For this review, take the finished solid that the model builds, in its own axes (mm). A direction names the side the tool comes from. Coordinates: 2 decimals unless noted, no trailing zeros. Order: outer loops, then holes, each group sorted by start corner. A loop starts at its lowest first (then second) coordinate and runs counter-clockwise, first axis right, second up. Notation, with made-up numbers: (51.5, 77.25) -> (87.5, 77.25) arc R19 ccw to (87.5, 108.25) -> close; hole circle Ø7 at (55, 85). An arc over 180 degrees is marked (long way). Return JSON: item names as keys, results as strings. Group by question number.
Item 1: Draft analysis for pull direction Y (two halves, no side actions). For faces 1 (the cylindrical face through (187.95, 4.47, -0.06)), 2 (the flat face through (101.23, 8.06, -0.42)), 3 (the flat face through (179.43, -2.385, -0.056)), state which applies: +Y half, -Y half, draft (parallel to the pull), parting line (faces both ways), or undercut.
Item 2: Machinability: for faces 4 (the flat face through (156, 54, 4)), 5 (the flat face through (192.854, 51, 0)), 6 (the flat face through (119.747, 51, 0)), 7 (the flat face through (99.28, -36.72, -0.06)), which of the approach directions +Z, -Z, +X, -X, +Y, -Y give a long, thin tool a straight path to every point of the face, cutting with its end or side? Answer none if there is none.
Item 3: Insertion check: pin 1 (1.5 mm diameter, centred on x = 123.5, z = -14, fed in from -Y); pin 2 (8 mm diameter, centred on x = 128.17, y = -49.49, fed in from +Z); pin 3 (11 mm diameter, centred on x = 166.5, y = 54, fed in from -Z); pin 4 (4.5 mm diameter, centred on x = 136.48, y = 50.87, fed in from -Z). Each pin has a flat end and moves straight along its axis. Give the tip position at first contact, or say it passes through.
Item 4: For line 1 along Z through (x, y) = (215.5, 24); line 2 along Y through (x, z) = (108, -22.5); line 3 along Y through (x, z) = (226, 21), list the stretches that pass through material, from the lowest coordinate up.
Item 5: Take a section at A-A (y = -10.5). Write out the cut boundary in (x, z).
```python
from build123d import *

# Parameters (mm, degrees)
RIGHT_MAIN_DEPTH    = 30
SKETCH2_R           = 2.5625
SKETCH2_R_2         = 2.563
RIGHTSCREWS_DEPTH   = 4
LEFT_MAIN_START     = -30
LEFT_MAIN_DEPTH     = 30
BOSS_EXTRUDE4_START = -4
LEFTSCRWS_R         = 2.5625
LEFTSCRWS_R_2       = 2.563
BOSS_EXTRUDE4_DEPTH = 4


with BuildPart() as part:
    # Sketch1 → right_main (new body)
    with BuildSketch(Plane.XY):
        with BuildLine():
            Line((107.405043491, 43.874842), (94.874715104, -28.778692489))
            add(Edge.make_bspline(
                [(94.874715104, -28.778692489), (125.81929731, -36.765852729), (149.855864514, -58.067716007)],
                knots=[0, 0, 0, 1, 1, 1], degree=2))
            Line((149.855864514, -58.067716007), (149.855864514, 43.874842))
            Line((149.855864514, 43.874842), (107.405043491, 43.874842))
        make_face()
        Polygon((149.855864514, 43.874842), (149.855864514, 28.52351163), (234.383754043, 28.52351163), (234.383754043, 43.874842), (192.853964769, 43.874842), align=None)
        with BuildLine():
            Line((149.855864514, 28.52351163), (149.855864514, -58.067716007))
            ThreePointArc((149.855864514, -58.067716007), (156.250771623, -25.404082318), (174.491218383, 2.436426025))
            ThreePointArc((174.491218383, 2.436426025), (201.883813055, 21.342868309), (234.383754043, 28.52351163))
            Line((234.383754043, 28.52351163), (149.855864514, 28.52351163))
        make_face()
    extrude(amount=RIGHT_MAIN_DEPTH)

    # Sketch2 → rightScrews (add)
    # profile 1 of 3: a face of its own
    with BuildSketch(Plane.XY):
        Polygon((119.747446117, 43.874842), (149.855864514, 43.874842), (192.853964769, 43.874842), (192.853964769, 57.874842), (119.747446117, 57.874842), align=None)
        with Locations((136.47520886, 50.874842)):
            Circle(SKETCH2_R, mode=Mode.SUBTRACT)
        with Locations((156.47520886, 50.874842)):
            Circle(SKETCH2_R, mode=Mode.SUBTRACT)
        with Locations((176.47520886, 50.874842)):
            Circle(SKETCH2_R, mode=Mode.SUBTRACT)
    # profile 2 of 3: a face of its own
    with BuildSketch(Plane.XY):
        with BuildLine():
            ThreePointArc((234.383754043, 28.52351163), (201.883813055, 21.342868309), (174.491218383, 2.436426025))
            Line((174.491218383, 2.436426025), (184.509352234, -7.342990836))
            add(Edge.make_bspline(
                [(184.509352234, -7.342990836), (204.930565052, 17.078226951), (234.383754043, 28.52351163)],
                knots=[0, 0, 0, 1, 1, 1], degree=2))
        make_face()
        with Locations((185.50732181, 3.700386733)):
            Circle(SKETCH2_R_2, mode=Mode.SUBTRACT)
    # profile 3 of 3: a face of its own
    with BuildSketch(Plane.XY):
        with BuildLine():
            Line((130.072927577, -58.067716007), (149.855864514, -58.067716007))
            add(Edge.make_bspline(
                [(101.184495321, -30.567929509), (128.298436124, -38.962933352), (149.855864514, -58.067716007)],
                knots=[0.103140303, 0.103140303, 0.103140303, 1, 1, 1], degree=2))
            Line((101.184495321, -30.567929509), (97.320282555, -43.048452225))
            Line((97.320282555, -43.048452225), (130.072927577, -58.067716007))
        make_face()
        with Locations((128.167744084, -49.493161828)):
            Circle(SKETCH2_R, mode=Mode.SUBTRACT)
        with Locations((109.079068542, -40.739735867)):
            Circle(SKETCH2_R, mode=Mode.SUBTRACT)
    extrude(amount=RIGHTSCREWS_DEPTH)

    # Sketch3 → left_main (add)
    with BuildSketch(Plane.XY.offset(LEFT_MAIN_START)):
        Polygon((149.855864514, 43.874842), (149.855864514, 28.52351163), (234.383754043, 28.52351163), (234.383754043, 43.874842), (192.853964769, 43.874842), align=None)
        with BuildLine():
            Line((107.405043491, 43.874842), (94.874715104, -28.778692489))
            add(Edge.make_bspline(
                [(94.874715104, -28.778692489), (125.81929731, -36.765852729), (149.855864514, -58.067716007)],
                knots=[0, 0, 0, 1, 1, 1], degree=2))
            Line((149.855864514, -58.067716007), (149.855864514, 43.874842))
            Line((149.855864514, 43.874842), (107.405043491, 43.874842))
        make_face()
        with BuildLine():
            Line((149.855864514, 28.52351163), (149.855864514, -58.067716007))
            ThreePointArc((149.855864514, -58.067716007), (156.250771623, -25.404082318), (174.491218383, 2.436426025))
            ThreePointArc((174.491218383, 2.436426025), (201.883813055, 21.342868309), (234.383754043, 28.52351163))
            Line((234.383754043, 28.52351163), (149.855864514, 28.52351163))
        make_face()
    extrude(amount=LEFT_MAIN_DEPTH)

    # leftScrws → Boss-Extrude4 (add)
    # profile 1 of 3: a face of its own
    with BuildSketch(Plane.XY.offset(BOSS_EXTRUDE4_START)):
        Polygon((119.747446117, 43.874842), (149.855864514, 43.874842), (192.853964769, 43.874842), (192.853964769, 57.874842), (119.747446117, 57.874842), align=None)
        with Locations((136.47520886, 50.874842)):
            Circle(LEFTSCRWS_R, mode=Mode.SUBTRACT)
        with Locations((156.47520886, 50.874842)):
            Circle(LEFTSCRWS_R, mode=Mode.SUBTRACT)
        with Locations((176.47520886, 50.874842)):
            Circle(LEFTSCRWS_R, mode=Mode.SUBTRACT)
    # profile 2 of 3: a face of its own
    with BuildSketch(Plane.XY.offset(BOSS_EXTRUDE4_START)):
        with BuildLine():
            Line((130.072927577, -58.067716007), (149.855864514, -58.067716007))
            add(Edge.make_bspline(
                [(101.184495321, -30.567929509), (128.298436124, -38.962933352), (149.855864514, -58.067716007)],
                knots=[0.103140303, 0.103140303, 0.103140303, 1, 1, 1], degree=2))
            Line((101.184495321, -30.567929509), (97.320282555, -43.048452225))
            Line((97.320282555, -43.048452225), (130.072927577, -58.067716007))
        make_face()
        with Locations((128.167744084, -49.493161828)):
            Circle(LEFTSCRWS_R, mode=Mode.SUBTRACT)
        with Locations((109.079068542, -40.739735867)):
            Circle(LEFTSCRWS_R, mode=Mode.SUBTRACT)
    # profile 3 of 3: a face of its own
    with BuildSketch(Plane.XY.offset(BOSS_EXTRUDE4_START)):
        with BuildLine():
            ThreePointArc((234.383754043, 28.52351163), (201.883813055, 21.342868309), (174.491218383, 2.436426025))
            Line((174.491218383, 2.436426025), (184.509352234, -7.342990836))
            add(Edge.make_bspline(
                [(184.509352234, -7.342990836), (204.930565052, 17.078226951), (234.383754043, 28.52351163)],
                knots=[0, 0, 0, 1, 1, 1], degree=2))
        make_face()
        with Locations((185.50732181, 3.700386733)):
            Circle(LEFTSCRWS_R_2, mode=Mode.SUBTRACT)
    extrude(amount=BOSS_EXTRUDE4_DEPTH)


solid = part.part
```
Findings below:
{
 "1": {"face 1": "undercut", "face 2": "+Y half", "face 3": "-Y half"},
 "2": {"face 4": "+Z, +X, -X, +Y", "face 5": "+Z, -Z, +X, +Y", "face 6": "+Z, -Z, -X, +Y", "face 7": "+Z, -Z, -X"},
 "3": {"pin 1": "stops at y = -40.18", "pin 2": "stops at z = 4", "pin 3": "stops at z = -4", "pin 4": "passes through"},
 "4": {"line 1": "z = -4 to 4", "line 2": "y = -32.88 to 43.87", "line 3": "y = 27.91 to 43.87"},
 "5": {"outline": "(98.03, -30) -> (164.09, -30) -> (164.09, 30) -> (98.03, 30) -> close"}
}
